Source: CAD feature listing. Evaluate the final solid. Frame: model axes, mm. A direction names the side the tool comes from. Give positions to 0.01 mm unless a question says otherwise; leave off trailing zeros. Write each loop counter-clockwise with the first axis right and the second up, starting at its lowest first coordinate (ties: lowest second). Pieces come first, ordered by that corner, then holes. Notation, with made-up numbers: (-6.5, -39.75) -> (33.5, -39.75) arc R16 cw to (33.5, -11.75) -> close; hole circle Ø5 at (-13, 53.5). An arc over 180 degrees is marked (long way). Use a Markdown table: item, result. Add a question column.
Autodesk Inventor part; units mm, degrees
ref_plane "YZ Plane" through (0, 0, 0) normal (1, 0, 0) x (0, 1, 0)
ref_plane "XZ Plane" through (0, 0, 0) normal (0, 1, 0) x (-1, 0, 0)
ref_plane "XY Plane" through (0, 0, 0) normal (0, 0, 1) x (1, 0, 0)
sketch "Sketch1" plane through (0, 0, 0) normal (0, 0, 1) x (1, 0, 0)
  point P0 (0, 0)
sketch "Sketch2" plane through (0, 0, 0) normal (0, 0, 1) x (1, 0, 0)
  line L0 (0, 0) -> (0, 131)
  line L1 (0, 131) -> (14, 131)
  line L2 (14, 131) -> (14, 0)
  line L3 (0, 0) -> (-4, 0)
  line L4 (14, 0) -> (18, 0)
  line L5 (18, 0) -> (18, -10)
  line L6 (18, -10) -> (-4, -10)
  line L7 (-4, -10) -> (-4, 0)
  dimension "d0" = 14
  dimension "d17" = 4
  dimension "d18" = 10
  dimension "d19" = 4
  dimension "d38" = 131
  dimension "d39" = 131
extrude "Extrusion1" add sketch "Sketch2" along normal blind 10
sketch "Sketch4" plane through (14, 0, 0) normal (1, 0, 0) x (0, 0, -1)
  line L0 (0, 131) -> (-10, 131)
  arc A0 (0, 131) -> (-10, 131) centre (-5, 131) ccw
  line L1 (0, 0) -> (-10, 0)
  arc A1 (-10, 0) -> (0, 0) centre (-5, 0) ccw
  dimension "d4" = 5
  dimension "d5" = 5
extrude "Extrusion2" add sketch "Sketch4" against normal blind 14 contours L0 A0
sketch "Sketch8" plane through (18, -10, 0) normal (1, 0, 0) x (0, 0, -1)
  circle A0 centre (-5, 5) radius 2.25
  line L0 (0, 0) -> (0, 10)
  line L1 (0, 0) -> (-10, 0)
  dimension "d21" = 4.5
  dimension "d22" = 5
  dimension "d23" = 5
extrude "Extrusion6" cut sketch "Sketch8" against normal blind 22
fillet "Fillet1" radius 5 1 edges at (7, -10, 10)
fillet "Fillet2" radius 5 1 edges at (7, -10, 0)
sketch "Sketch10" plane through (14, 0, 10) normal (1, 0, 0) x (0, 0, -1)
  circle A0 centre (5, 131) radius 2.25
  line L0 (10, 0) -> (10, 131)
  arc A1 (10, 131) -> (0, 131) centre (5, 131) ccw
  dimension "d28" = 4.5
  dimension "d29" = 5
  dimension "d30" = 0
extrude "Extrusion7" cut sketch "Sketch10" against normal blind 14
sketch "Sketch11" plane through (0, 0, 0) normal (0, 0, -1) x (-1, 0, 0)
  line L0 (-4, 0) -> (-10, 0)
  line L1 (-10, 0) -> (-10, -10)
  line L2 (4, -10) -> (-18, -10)
  line L3 (-4, -10) -> (-4, 0)
  line L4 (-14, 0) -> (-14, 131)
  point P0 (0, 0)
  dimension "d33" = 4
  dimension "d34" = 4
  dimension "d35" = 6
extrude "Extrusion8" cut sketch "Sketch11" against normal blind 10
sketch "Sketch20" plane through (0, 0, 10) normal (0, 0, 1) x (1, 0, 0)
  line L0 (4, -5) -> (4, 0)
  line L1 (4, 0) -> (0, -5)
  line L2 (-4, -5) -> (4, -5)
  line L3 (4, -5) -> (4, -10)
  line L4 (0, -5) -> (4, -5)
  line L5 (4, 0) -> (4, -5)
  point P0 (0, 0)
extrude "Extrusion16" cut sketch "Sketch20" against normal blind 10
sketch "Sketch21" plane through (0, 0, 10) normal (0, 0, 1) x (1, 0, 0)
  line L0 (0, -5) -> (4, 0)
  line L1 (4, -5) -> (4, -10)
  line L2 (0, -5) -> (4, -5)
  line L3 (-4, -10) -> (4, -10)
  line L4 (4, -10) -> (0, -10)
  line L5 (-4, -5) -> (0, -5)
  line L6 (0, -5) -> (0, -10)
  line L7 (4, -5) -> (4, -10)
  point P0 (0, 0)
extrude "Extrusion17" cut sketch "Sketch21" against normal blind 10
sketch "Sketch22" plane through (0, 0, 10) normal (0, 0, 1) x (1, 0, 0)
  line L0 (10, -5) -> (10, 0)
  line L1 (10, 0) -> (14, -5)
  line L2 (10, -5) -> (18, -5)
  line L3 (10, 0) -> (10, -5)
  line L4 (10, -5) -> (14, -5)
  point P0 (0, 0)
extrude "Extrusion18" cut sketch "Sketch22" against normal blind 10
sketch "Sketch23" plane through (0, 0, 10) normal (0, 0, 1) x (1, 0, 0)
  line L0 (10, -10) -> (10, -5)
  line L1 (18, -5) -> (14, -5)
  line L2 (10, -5) -> (14, -5)
  line L3 (14, -5) -> (14, -10)
  line L4 (10, -10) -> (18, -10)
  line L5 (10, -5) -> (10, -10)
  line L6 (10, -10) -> (14, -10)
  point P0 (0, 0)
extrude "Extrusion19" cut sketch "Sketch23" against normal blind 10
sketch "Sketch24" plane through (0, 0, 10) normal (0, 0, 1) x (1, 0, 0)
  line L0 (4, 0) -> (10, 0)
  line L1 (4, 0) -> (4.8, 1)
  line L2 (0, -5) -> (4, 0)
  line L3 (4.8, 1) -> (9.2, 1)
  line L4 (14, -5) -> (10, 0)
  line L5 (9.2, 1) -> (10, 0)
  point P0 (0, 0)
  dimension "d66" = 1
extrude "Extrusion20" cut sketch "Sketch24" against normal blind 10
sketch "Sketch25" plane through (0, 0, 10) normal (0, 0, 1) x (1, 0, 0)
  line L0 (5, 116) -> (9, 116)
  line L1 (9, 116) -> (9, 16)
  line L2 (9, 16) -> (5, 16)
  line L3 (5, 16) -> (5, 116)
  line L4 (14, 0) -> (14, 131)
  line L5 (14, 131) -> (0, 131)
  line L6 (4.8, 1) -> (9.2, 1)
  line L7 (0, 131) -> (0, 0)
  dimension "d82" = 5
  dimension "d84" = 4
  dimension "d85" = 100
  dimension "d86" = 15
extrude "Extrusion21" cut sketch "Sketch25" against normal blind 10
properties part number "Rod"
(1) Material intervals for L1, parallel to Y at x = 6.5, z = 5; L2, parallel to X at y = 112.5, z = 6.5; L3, parallel to Y at x = -2.3, z = 5, sorted ascending.
(2) Cut plane A-A on y = 21.5. Return the cut outline in (x, z).
(3) Access query for faces 5 (the flat face through (2.4, -2, 5.1)), 6 (the cylindrical face through (7, 136, 5)), 7 (the flat face through (5, 65, 5)), 8 (the flat face through (16, 0, 5)). Directions: +Z, -Z, +X, -X, +Y, -Y. A direction counts if a zero-diameter tool reaches every point of the face in a straight line with its end or side. Return the directions, or none.
(4) Cut plane B-B on z = 8.5. Return the cut outline in (x, y).
(5) Cut plane C-C on y = 122.5. Return the cut outline in (x, z).
(6) Mould query, pull axis X, two halves, no side actions, for faces 1 (the flat face through (-4, -2.8, 6)), 2 (the flat face through (7, 116, 5)), 3 (the flat face through (18, -2.7, 6)), 4 (the flat face through (-2, 0, 5)). Classes: +X half, -X half, draft (parallel to the pull), parting line (faces both ways), or undercut.
(7) First-contact query: pin 1 Ø1.5 at (y, z) = (-7, 5.5) entering from +X; pin 2 Ø4 at (y, z) = (45, 1.5) entering from -X; pin 3 Ø5 at (y, z) = (77.5, 4) entering from +X; pin 4 Ø2 at (x, z) = (7, 6.5) entering from -Y. Flat tips, straight axial feed; report the tip coordinate or a pass-through.
Output:
| question | item | result |
|---|---|---|
| 1 | L1 | 1 to 16, 116 to 128.75, 133.25 to 136 |
| 1 | L2 | 0 to 5, 9 to 14 |
| 1 | L3 | -10 to -7.25, -2.75 to 0 |
| 2 | outline | (0, 0) -> (5, 0) -> (5, 10) -> (0, 10) -> close; (9, 0) -> (14, 0) -> (14, 10) -> (9, 10) -> close |
| 3 | face 5 | +Z, -Z, -Y |
| 3 | face 6 | +X, -X, +Y |
| 3 | face 7 | +Z, -Z |
| 3 | face 8 | +Z, -Z, +X, +Y |
| 4 | outline | (-4, -8.57) -> (0, -8.57) -> (0, -5) -> (4.8, 1) -> (9.2, 1) -> (14, -5) -> (14, -8.57) -> (18, -8.57) -> (18, 0) -> (14, 0) -> (14, 134.57) -> (0, 134.57) -> (0, 0) -> (-4, 0) -> close; hole (5, 16) -> (9, 16) -> (9, 116) -> (5, 116) -> close |
| 5 | outline | (0, 0) -> (14, 0) -> (14, 10) -> (0, 10) -> close |
| 6 | face 1 | -X half |
| 6 | face 2 | undercut |
| 6 | face 3 | +X half |
| 6 | face 4 | draft |
| 7 | pin 1 | x = 18 |
| 7 | pin 2 | x = 0 |
| 7 | pin 3 | x = 14 |
| 7 | pin 4 | y = 1 |
